Source: CAD feature listing. Evaluate the final solid. Frame: model axes, mm. A direction names the side the tool comes from. Give positions to 0.01 mm unless a question says otherwise; leave off trailing zeros. Order: outer loops, then holes, each group sorted by start corner. A loop starts at its lowest first (then second) coordinate and runs counter-clockwise, first axis right, second up. Notation, with made-up numbers: M -12,16.25 L -5,16.25 A10 ccw -5,21.25 Z; hole C 75.5,-29 d2. An arc over 180 degrees is marked long. One line per question, with ' | ' between items. Start each with the question number.
Autodesk Inventor part; units mm, degrees
ref_plane "YZ Plane" through (0, 0, 0) normal (1, 0, 0) x (0, 1, 0)
ref_plane "XZ Plane" through (0, 0, 0) normal (0, 1, 0) x (-1, 0, 0)
ref_plane "XY Plane" through (0, 0, 0) normal (0, 0, 1) x (1, 0, 0)
sketch "Skizze1" plane through (0, 0, 0) normal (1, 0, 0) x (0, 1, 0)
  circle A0 centre (0, 0) radius 18.5
  dimension "d0" = 37
extrude "Extrusion1" add sketch "Skizze1" along normal blind 26.5
sketch "Skizze2" plane through (26.5, 0, 0) normal (1, 0, 0) x (0, 0, -1)
  circle A0 centre (0, 0) radius 16.3
  dimension "d3" = 32.6
extrude "Extrusion2" add sketch "Skizze2" along normal blind 23
sketch "Skizze3" plane through (49.5, 0, 0) normal (1, 0, 0) x (0, 0, -1)
  circle A0 centre (0, 0) radius 4
  dimension "d6" = 8
extrude "Extrusion3" add sketch "Skizze3" along normal blind 3
sketch "Skizze4" plane through (0, 0, 0) normal (-1, 0, 0) x (0, 0, 1)
  line L0 (-25.9, 0) -> (25.9, 0)
  line L1 (0, 25.9) -> (0, -25.9)
  circle A0 centre (7, 0) radius 6
  point P0 (0, 0)
  dimension "d9" = 12
  dimension "d10" = 7
extrude "Extrusion4" add sketch "Skizze4" along normal blind 6
sketch "Skizze5" plane through (-6, 0, 7) normal (-1, 0, 0) x (0, 0, 1)
  circle A0 centre (0, 0) radius 6
  circle A1 centre (0, 0) radius 3
  point P0 (-7, 0)
  dimension "d13" = 6
extrude "Extrusion5" add sketch "Skizze5" along normal blind 15 contours A1
sketch "Skizze6" plane through (0, 0, 0) normal (-1, 0, 0) x (0, 0, 1)
  line L0 (-25.9, 0) -> (25.9, 0)
  line L1 (0, 25.9) -> (0, -25.9)
  circle A0 centre (0, 0) radius 15.4 construction
  point P0 (0, 15.4)
  point P1 (-13.3368, 7.7)
  point P2 (-13.3368, -7.7)
  point P3 (0, -15.4)
  point P4 (13.3368, -7.7)
  point P5 (13.3368, 7.7)
  dimension "d16" = 30.8
  dimension "d19" = 360
hole "Bohrung1" at (0, 15.4, 0) at (0, 7.7, -13.3368) at (0, -7.7, -13.3368) at (0, -15.4, 0) at (0, -7.7, 13.3368) at (0, 7.7, 13.3368) direction (1, 0, 0) diameter 2.459 depth 6 tip angle 118
properties part number "V-TEC 12V Mini 37D DC"
Item 1: Cut plane D-D on x = 35.5. Return the cut outline in (y, z), and give its area (3 significant figures).
Item 2: Cut plane A-A on y = 2. Return the cut outline in (x, z).
Item 3: Cut plane C-C on z = 7. Return the cut outline in (x, y), and give its area (3 significant figures).
Item 4: Line query: line 1 (Z direction, x = 2, y = 7); line 2 (X direction, y = 16.5, z = 5); line 3 (Y direction, x = 4, z = 14). Output: solid intervals per line, ascending.
Item 5: Cut plane B-B on x = 8.5. Return the cut outline in (y, z), and give its area (3 significant figures).
Item 6: Pin query (flat end, axial travel): pin 1 Ø1 at (x, z) = (30, -14) entering from -Y; pin 2 Ø10 at (y, z) = (-11.5, 6) entering from -X; pin 3 Ø1.5 at (y, z) = (7.7, 13.34) entering from -X. Return the tip coordinate at first contact, or that it passes through.
Item 7: Reachability of faces 1 (the cylindrical face through (3.042, -8.531, -14.243)), 2 (the flat face through (-21, 0, 7)), 3 (the cylindrical face through (50.979, 3.905, 0.867)) from +Z, -Z, +X, -X, +Y, -Y: full face, straight path, thin tool, end or side. Return the list, or none.
Item 8: Mould query, pull axis Z, two halves, no side actions, for faces 4 (the flat face through (52.5, 0, 0)), 5 (the cylindrical face through (3.042, -14.652, -0.976)), 6 (the cylindrical face through (-3, 0, 1)). Classes: pulls with the +Z half, pulls with the -Z half, needs draft (parallel to the pull), parting line crosses it, or undercut.
Results are:
1) outline: C 0,0 d32.6 | area: 835 mm2
2) outline: M -21,4.76 L -6,4.76 L -6,1.34 L 0,1.34 L 0,-18.39 L 26.5,-18.39 L 26.5,-16.18 L 49.5,-16.18 L 49.5,-3.46 L 52.5,-3.46 L 52.5,3.46 L 49.5,3.46 L 49.5,16.18 L 26.5,16.18 L 26.5,18.39 L 0,18.39 L 0,12.66 L -6,12.66 L -6,9.24 L -21,9.24 Z
3) outline: M -21,-3 L -6,-3 L -6,-6 L 0,-6 L 0,-17.12 L 26.5,-17.12 L 26.5,-14.72 L 49.5,-14.72 L 49.5,14.72 L 26.5,14.72 L 26.5,17.12 L 0,17.12 L 0,6 L -6,6 L -6,3 L -21,3 Z | area: 1,750 mm2
4) line 1: z = -17.12 to -14.35, -12.33 to 12.33, 14.35 to 17.12 | line 2: x = 0 to 26.5 | line 3: y = -12.09 to -8.74, -6.66 to 6.66, 8.74 to 12.09
5) outline: C 0,0 d37 | area: 1,080 mm2
6) pin 1: stops at y = -9.13 | pin 2: stops at x = 0 | pin 3: stops at x = 6.29
7) face 1: -X | face 2: +Z, -Z, -X, +Y, -Y | face 3: +X
8) face 4: needs draft | face 5: undercut | face 6: parting line crosses it
